from build123d import *

# Parameters (mm, degrees)
SKIZZE1_R                        = 4
AUFSATZ_LINEAR_AUSTRAGEN1_DEPTH  = 21.6
F_3_2_3_2_DURCHMESSER_BOHRUNG1_D = 3.2
FASE1_SIZE                       = 0.4


with BuildPart() as part:
    # Skizze1 → Aufsatz-Linear austragen1 (new body)
    with BuildSketch(Plane(origin=(0, 0, 0), x_dir=(0, 0, -1), z_dir=(1, 0, 0))):
        with Locations(Location((0, 0, 0), (0, 0, 180))):
            Circle(SKIZZE1_R)
    extrude(amount=AUFSATZ_LINEAR_AUSTRAGEN1_DEPTH)

    # Ø3.2 (3.2) Durchmesser Bohrung1 (through all)
    with Locations(Plane(origin=(21.6, 0, 0), x_dir=(0, 0, -1), z_dir=(1, 0, 0))):
        with Locations((0, 0)):
            Hole(F_3_2_3_2_DURCHMESSER_BOHRUNG1_D / 2)

    # Fase1
    fase1_edges = [part.edges().sort_by_distance(p)[0] for p in [
        (21.6, 0, -1.6),
        (0, 0, -1.6),
    ]]
    chamfer(fase1_edges, length=FASE1_SIZE)


solid = part.part
For this review, take the finished solid that the model builds, in its own axes (mm). Round coordinates to 2 decimals unless told otherwise and drop trailing zeros. Order: outer loops, then holes, each group sorted by start corner. A loop starts at its lowest first (then second) coordinate and runs counter-clockwise, first axis right, second up. Notation, with made-up numbers: (-38, 60) -> (16, 60) arc R24 ccw to (16, 79) -> close; hole circle Ø7 at (87, 26). An arc over 180 degrees is marked (long way). Put each result on its own line as item: value.
Q1. Mouldability with a two-part tool opening along Z and no side actions: class faces 1 (the flat face through (0, 1, -2)), 2 (the cylindrical face through (10.65, -0.97, -1.27)), 3 (the cylindrical face through (10.649, 3.905, -0.867)) as pulls with the +Z half, pulls with the -Z half, needs draft (parallel to the pull), parting line crosses it, or undercut.
Check result:
face 1: needs draft
face 2: undercut
face 3: parting line crosses it
Q2. Add section A-A on z = 0. Write out the cut boundary in (x, y), plus the area to 3 significant figures.
Check result:
outline: (0, -4) -> (21.6, -4) -> (21.6, -2) -> (21.2, -1.6) -> (0.4, -1.6) -> (0, -2) -> close; (0, 2) -> (0.4, 1.6) -> (21.2, 1.6) -> (21.6, 2) -> (21.6, 4) -> (0, 4) -> close
area: 103 mm2
Q3. Add section D-D on z = -3.5. Write out the cut boundary in (x, y).
Check result:
outline: (0, -1.94) -> (21.6, -1.94) -> (21.6, 1.94) -> (0, 1.94) -> close
Q4. For probe 1 along Y at (x, z) = (11.25, 0); probe 2 along Z at (x, y) = (5, 1); probe 3 along Z at (x, y) = (18.5, 0.5), list the stretches that pass through material, from the lowest coordinate up. Write a range as [from, to].
Check result:
probe 1: [-4, -1.6], [1.6, 4]
probe 2: [-3.87, -1.25], [1.25, 3.87]
probe 3: [-3.97, -1.52], [1.52, 3.97]
Q5. Insertion check: pin 1 Ø3.5 at (y, z) = (0, 0) entering from -X; pin 2 Ø4 at (x, y) = (8, 3) entering from +Z; pin 3 Ø2 at (x, z) = (16.5, -2.5) entering from +Y. Each pin has a flat end and moves straight along its axis. Give the tip position at first contact, or say it passes through.
Check result:
pin 1: x = 0.25
pin 2: z = 3.87
pin 3: y = 3.71
Q6. Add section B-B on x = 18.25. Write out the cut boundary in (y, z).
Check result:
outline: circle Ø8 at (0, 0); hole circle Ø3.2 at (0, 0)
Q7. Add section C-C on y = 3. Write out the cut boundary in (x, z), plus the area to 3 significant figures.
Check result:
outline: (0, -2.65) -> (21.6, -2.65) -> (21.6, 2.65) -> (0, 2.65) -> close
area: 114 mm2
